```python
from build123d import *

# Parameters (mm, degrees)
BOSS_EXTRUDE1_DEPTH = 30
CUT_EXTRUDE1_DEPTH  = 10
CUT_EXTRUDE2_DEPTH  = 10
SKETCH5_R           = 2.25
CUT_EXTRUDE3_DEPTH  = 46
SKETCH6_R           = 2.25
CUT_EXTRUDE4_DEPTH  = 10


with BuildPart() as part:
    # Sketch1 → Boss-Extrude1 (new body)
    with BuildSketch(Plane.XY):
        Polygon((0, 0), (0, 6), (7, 6), (16, 15), (56, 15), (56, 45), (101, 45), (101, 35), (66, 35), (66, 5), (12, 5), (7, 0), align=None)
    extrude(amount=BOSS_EXTRUDE1_DEPTH)

    # Sketch2 → Cut-Extrude1 (cut)
    with BuildSketch(Plane.XY.offset(30)):
        Polygon((26, 15), (26, 5), (66, 5), (66, 35), (101, 35), (101, 45), (56, 45), (56, 15), align=None)
    extrude(amount=-CUT_EXTRUDE1_DEPTH, mode=Mode.SUBTRACT)

    # Sketch4 → Cut-Extrude2 (cut)
    with BuildSketch(Plane(origin=(0, 0, 0), x_dir=(-1, 0, 0), z_dir=(0, 0, -1))):
        Polygon((-66, 5), (-26, 5), (-26, 15), (-56, 15), (-56, 45), (-101, 45), (-101, 35), (-66, 35), align=None)
    extrude(amount=-CUT_EXTRUDE2_DEPTH, mode=Mode.SUBTRACT)

    # Sketch5 → Cut-Extrude3 (cut, through all)
    with BuildSketch(Plane(origin=(0, 45, 0), x_dir=(1, 0, 0), z_dir=(0, 1, 0))):
        with Locations((94.248435015, -15)):
            Circle(SKETCH5_R)
    extrude(amount=-CUT_EXTRUDE3_DEPTH, mode=Mode.SUBTRACT)

    # Sketch6 → Cut-Extrude4 (cut)
    with BuildSketch(Plane(origin=(0, 6, 0), x_dir=(1, 0, 0), z_dir=(0, 1, 0))):
        with Locations((3.5, -6)):
            Circle(SKETCH6_R)
        with Locations((3.5, -24)):
            Circle(SKETCH6_R)
    extrude(amount=-CUT_EXTRUDE4_DEPTH, mode=Mode.SUBTRACT)


solid = part.part
```
Read the model definition and answer for the solid it produces. Units are mm, in the model's axes. A direction names the side the tool comes from. Coordinates: 2 decimals unless noted, no trailing zeros. Loops run counter-clockwise (first coordinate to the right, second up) from the corner with the lowest first, then second, coordinate; pieces in that order, holes last. Notation, with made-up numbers: (81.25, 29) -> (137.25, 29) arc R30 cw to (137.25, 65) -> close; hole circle Ø3 at (-35.5, 70). An arc over 180 degrees is marked (long way). Return JSON: item names as keys, results as strings.
Item 1: Find section A-A (z = 15). Determine the outline of the cut face in (x, y), plus the area to 3 significant figures.
Answers:
{"outline": "(0, 0) -> (7, 0) -> (12, 5) -> (66, 5) -> (66, 35) -> (92, 35) -> (92, 45) -> (56, 45) -> (56, 15) -> (16, 15) -> (7, 6) -> (0, 6) -> close; (96.5, 35) -> (101, 35) -> (101, 45) -> (96.5, 45) -> close", "area": "1,210 mm2"}
Item 2: For a pull along X with two mould halves and no side action, classify faces 1 (the flat face through (66, 20, 15)), 2 (the cylindrical face through (3.012, 3.042, 26.196)), 3 (the flat face through (13, 8, 30)) as +X half, -X half, draft (parallel to the pull), parting line (faces both ways), or undercut.
Answers:
{"face 1": "+X half", "face 2": "undercut", "face 3": "draft"}
Item 3: Find section D-D (z = 2.75). Determine the outline of the cut face in (x, y), plus the area to 3 significant figures.
Answers:
{"outline": "(0, 0) -> (7, 0) -> (12, 5) -> (26, 5) -> (26, 15) -> (16, 15) -> (7, 6) -> (0, 6) -> close", "area": "204 mm2"}
Item 4: Find the intervals of material crossed by probe 1 along X at (y, z) = (40, 15); probe 2 along Z at (x, y) = (3.5, 3.2); probe 3 along Z at (x, y) = (29.5, 11), in increasing order.
Answers:
{"probe 1": "x = 56 to 92, 96.5 to 101", "probe 2": "z = 0 to 3.75, 8.25 to 21.75, 26.25 to 30", "probe 3": "z = 10 to 20"}
Item 5: For faces 4 (the flat face through (26, 10, 25)), 5 (the flat face through (84, 35, 15)), 6 (the flat face through (26, 10, 5)), 7 (the flat face through (56, 30, 15)), determine the directions among +Z, -Z, +X, -X, +Y, -Y from which every point of the face is accessible in a straight line to the end or side of a thin tool.
Answers:
{"face 4": "+Z, +X, +Y, -Y", "face 5": "+Z, -Z, +X, -Y", "face 6": "-Z, +X, +Y, -Y", "face 7": "+Z, -Z, -X, +Y"}
Item 6: Flat-ended cylindrical pins translate along their axes: P1, Ø5, axis at y = 30, z = 14, coming from the -X side; P2, Ø11, axis at x = 79.5, z = 17, coming from the -Y side; P3, Ø8, axis at y = 10, z = 26, coming from the +X side. Find the tip coordinate at first contact, or state that the pin passes through.
Answers:
{"P1": "stops at x = 56", "P2": "stops at y = 35", "P3": "stops at x = 26"}
Item 7: Find section C-C (y = 14). Determine the outline of the cut face in (x, z).
Answers:
{"outline": "(15, 0) -> (26, 0) -> (26, 10) -> (66, 10) -> (66, 20) -> (26, 20) -> (26, 30) -> (15, 30) -> close"}
Item 8: Find section B-B (y = 4). Determine the outline of the cut face in (x, z), plus the area to 3 significant figures.
Answers:
{"outline": "(0, 0) -> (11, 0) -> (11, 30) -> (0, 30) -> close; hole circle Ø4.5 at (3.5, 6); hole circle Ø4.5 at (3.5, 24)", "area": "298 mm2"}
